from build123d import *

# Parameters (mm, degrees)
SKETCH_R        = 2.25
SKETCH_R_2      = 11.25
SKETCH_R_3      = 1.75
PAD_DEPTH       = 14.3
POCKET_DEPTH    = 8.6
SKETCH004_R     = 2.25
POCKET003_DEPTH = 10
SKETCH005_R     = 4.05
POCKET004_DEPTH = 12
SKETCH006_R     = 3.75
POCKET005_DEPTH = 9.2


with BuildPart() as pocket005:
    # Sketch → Pad (new body)
    with BuildSketch(Plane.XY):
        Polygon((0, 0), (105, 0), (105, 62), (20, 62), (20, 42), (0, 42), align=None)
        with Locations((38, 10)):
            Circle(SKETCH_R, mode=Mode.SUBTRACT)
        with Locations((33, 35)):
            Circle(SKETCH_R, mode=Mode.SUBTRACT)
        with Locations((84, 21)):
            Circle(SKETCH_R_2, mode=Mode.SUBTRACT)
        with Locations((68.5, 36.5)):
            Circle(SKETCH_R_3, mode=Mode.SUBTRACT)
        with Locations((99.5, 36.5)):
            Circle(SKETCH_R_3, mode=Mode.SUBTRACT)
        with Locations((68.5, 5.5)):
            Circle(SKETCH_R_3, mode=Mode.SUBTRACT)
        with Locations((99.5, 5.5)):
            Circle(SKETCH_R_3, mode=Mode.SUBTRACT)
        with Locations((10, 30)):
            Circle(SKETCH_R, mode=Mode.SUBTRACT)
        with Locations((10, 15)):
            Circle(SKETCH_R, mode=Mode.SUBTRACT)
        with Locations((42, 52)):
            Circle(SKETCH_R, mode=Mode.SUBTRACT)
        with Locations((94, 52)):
            Circle(SKETCH_R, mode=Mode.SUBTRACT)
        with BuildLine():
            Line((58.75, 25), (58.75, 39.999999))
            ThreePointArc((58.75, 39.999999), (56.5, 42.25), (54.25, 39.999998))
            Line((54.25, 25.000001), (54.25, 39.999998))
            ThreePointArc((54.25, 25.000001), (56.5, 22.75), (58.75, 25))
        make_face(mode=Mode.SUBTRACT)
    extrude(amount=PAD_DEPTH)

    # Sketch001 → Pocket (cut)
    with BuildSketch(Plane.XY.offset(14.3)):
        with BuildLine():
            ThreePointArc((41.485277, 42), (39.015593, 44.209375), (35.999996, 45.583005))
            Line((35.999996, 67), (35.999996, 45.583005))
            Line((20, 67), (35.999996, 67))
            Line((20, -1), (20, 67))
            Line((20, -1), (48.252269, -1))
            Line((48.252269, 11), (48.252269, -1))
            Line((48.252269, 11), (70.252269, 11))
            ThreePointArc((70.252269, 11), (71.759618, 9.202833), (73.499996, 7.630258))
            Line((73.499996, 7.630258), (73.499996, -1))
            Line((73.499996, -1), (93.499996, -1))
            Line((93.499996, -1), (93.499996, 6.902128))
            ThreePointArc((93.499996, 6.902128), (95.574295, 8.548671), (97.367695, 10.497399))
            Line((105.499996, 10.497399), (97.367695, 10.497399))
            Line((105.499996, 30.497399), (105.499996, 10.497399))
            Line((98.099621, 30.497399), (105.499996, 30.497399))
            ThreePointArc((98.099621, 30.497399), (91.98574, 36.007594), (83.999996, 38))
            Line((83.999996, 38), (83.999996, 67))
            Line((83.999996, 67), (46.999996, 67))
            Line((46.999996, 67), (46.999996, 42))
            Line((41.485277, 42), (46.999996, 42))
        make_face()
    extrude(amount=-POCKET_DEPTH, mode=Mode.SUBTRACT)

    # Sketch004 → Pocket003 (cut)
    with BuildSketch(Plane.XY.offset(14.3)):
        with Locations((55, 5)):
            Circle(SKETCH004_R)
    extrude(amount=-POCKET003_DEPTH, mode=Mode.SUBTRACT)

    # Sketch005 → Pocket004 (cut)
    with BuildSketch(Plane.XZ):
        with Locations((13, 14.3)):
            Circle(SKETCH005_R)
    extrude(amount=-POCKET004_DEPTH, mode=Mode.SUBTRACT)

    # Sketch006 → Pocket005 (cut)
    with BuildSketch(Plane(origin=(0, 0, 0), x_dir=(1, 0, 0), z_dir=(0, 0, -1))):
        with Locations((10, -15)):
            Circle(SKETCH006_R)
        with Locations((10, -30)):
            Circle(SKETCH006_R)
        with Locations((42, -52)):
            Circle(SKETCH006_R)
        with Locations((94, -52)):
            Circle(SKETCH006_R)
    extrude(amount=-POCKET005_DEPTH, mode=Mode.SUBTRACT)


with BuildPart() as part_mirroring:
    # Part__Mirroring: instance of Pocket005
    add(pocket005.part.mirror(Plane(origin=(0, 0, 0), x_dir=(0, -1, 0), z_dir=(1, 0, 0))))


solid = part_mirroring.part
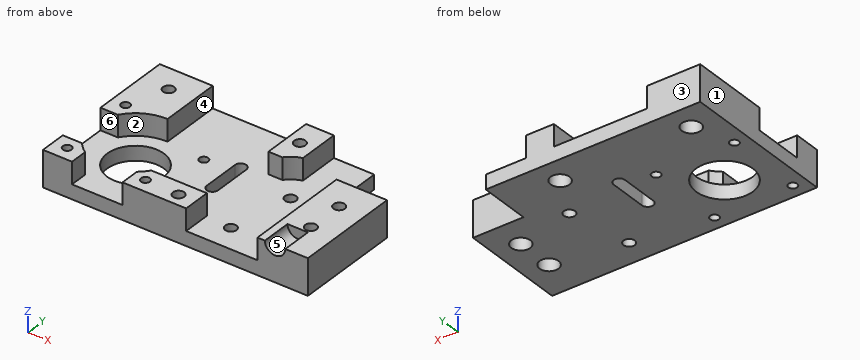
For this review, take the finished solid that the model builds, in its own axes (mm). Face numbers are marked on the shaded views. A direction names the side the tool comes from. Coordinates: 2 decimals unless noted, no trailing zeros. Order: outer loops, then holes, each group sorted by start corner. A loop starts at its lowest first (then second) coordinate and runs counter-clockwise, first axis right, second up. Notation, with made-up numbers: (6, -16) -> (52, -16) arc R17 cw to (52, -9) -> close; hole circle Ø7 at (64, -35.5). An arc over 180 degrees is marked (long way). Return JSON: item names as keys, results as strings.
1. We need section B-B on y = 52. Write out the cut boundary in (x, z), and give its area (3 significant figures).
Answer block:
{"outline": "(-105, 0) -> (-97.75, 0) -> (-97.75, 9.2) -> (-96.25, 9.2) -> (-96.25, 14.3) -> (-105, 14.3) -> close; (-91.75, 9.2) -> (-90.25, 9.2) -> (-90.25, 0) -> (-45.75, 0) -> (-45.75, 9.2) -> (-44.25, 9.2) -> (-44.25, 14.3) -> (-47, 14.3) -> (-47, 5.7) -> (-84, 5.7) -> (-84, 14.3) -> (-91.75, 14.3) -> close; (-39.75, 9.2) -> (-38.25, 9.2) -> (-38.25, 0) -> (-20, 0) -> (-20, 5.7) -> (-36, 5.7) -> (-36, 14.3) -> (-39.75, 14.3) -> close", "area": "576 mm²"}
2. The part is to be moulded in two halves that separate along X. For the marked faces 1, 2 and 3, say which applies: +X half, -X half, draft (parallel to the pull), parting line (faces both ways), or undercut.
Answer block:
{"face 1": "-X half", "face 2": "undercut", "face 3": "draft"}
3. For pin 1 Ø3.5 at (x, y) = (-94, 52) entering from +Z (1 decimal); pin 2 Ø4.5 at (x, z) = (-12.5, 12) entering from -Y; pin 3 Ø2.5 at (x, y) = (-55, 5) entering from +Z; pin 4 Ø3 at (y, z) = (26.5, 8.5) entering from -X, all flat-tipped, find the tip position at first contact; note any pin that passes through.
Answer block:
{"pin 1": "through", "pin 2": "y = 0", "pin 3": "z = 4.3", "pin 4": "x = -20"}
4. For line 1 (Y direction, x = -10, z = 11.75); line 2 (Y direction, x = -33, z = 3.4); line 3 (Y direction, x = -94, z = 11.55), list the stretches that pass through material, from the lowest coordinate up. Write a range as from..to.
Answer block:
{"line 1": "12..12.75, 17.25..27.75, 32.25..42", "line 2": "0..32.75, 37.25..62", "line 3": "0..7.25, 34.75..49.75, 54.25..62"}
5. We need section D-D on x = -68.5. Write out the cut boundary in (y, z).
Answer block:
{"outline": "(0, 0) -> (3.75, 0) -> (3.75, 14.3) -> (0, 14.3) -> close; (7.25, 0) -> (34.75, 0) -> (34.75, 5.7) -> (11, 5.7) -> (11, 14.3) -> (7.25, 14.3) -> close; (38.25, 0) -> (62, 0) -> (62, 5.7) -> (38.25, 5.7) -> close"}
6. We need section C-C on x = -33. Write out the cut boundary in (y, z).
Answer block:
{"outline": "(0, 0) -> (32.75, 0) -> (32.75, 5.7) -> (0, 5.7) -> close; (37.25, 0) -> (62, 0) -> (62, 5.7) -> (37.25, 5.7) -> close"}
7. Machinability: for the marked faces 4, 5 and 6, which of the approach directions +Z, -Z, +X, -X, +Y, -Y give a long, thin tool a straight path to every point of the face, cutting with its end or side? Answer none if there is none.
Answer block:
{"face 4": "+Z, +Y, -Y", "face 5": "+Z, -Y", "face 6": "+Z, -X"}
8. We need section A-A on z = 7. State how many separate pieces and enclosed holes the cut face has, and give its area (3 significant figures).
Answer block:
{"separate pieces": "5", "enclosed holes": "8", "area": "1,800 mm²"}
